Could you check a few things on this model? Use its own coordinates, in mm. Round coordinates to 2 decimals unless told otherwise and drop trailing zeros. Write each loop counter-clockwise with the first axis right and the second up, starting at its lowest first coordinate (ties: lowest second). Pieces come first, ordered by that corner, then holes. Notation, with made-up numbers: (26.5, 9.25) - (55.5, 9.25) arc R16 cw to (55.5, 17.25) - close; hole circle Ø5 at (2.5, 71). An arc over 180 degrees is marked (long way). Put each result on its own line as item: value.
from build123d import *

# Parameters (mm, degrees)
SKETCH1_R           = 3
SKETCH1_R_2         = 11.5
BOSS_EXTRUDE1_DEPTH = 4.7625


with BuildPart() as part:
    # Sketch1 → Boss-Extrude1 (new body)
    with BuildSketch(Plane.XY):
        Polygon((21.936631743, 65.154612456), (-64.58116939, 4.790688487), (-30.249253249, -44.416216862), (56.268547885, 15.947707107), align=None)
        with Locations(Location((-22.811758645, -2.646806117, 0), (0, 0, 180))):
            Circle(SKETCH1_R, mode=Mode.SUBTRACT)
        with Locations(Location((22.800025974, 29.176775421, 0), (0, 0, 180))):
            Circle(SKETCH1_R_2, mode=Mode.SUBTRACT)
    extrude(amount=BOSS_EXTRUDE1_DEPTH)


solid = part.part
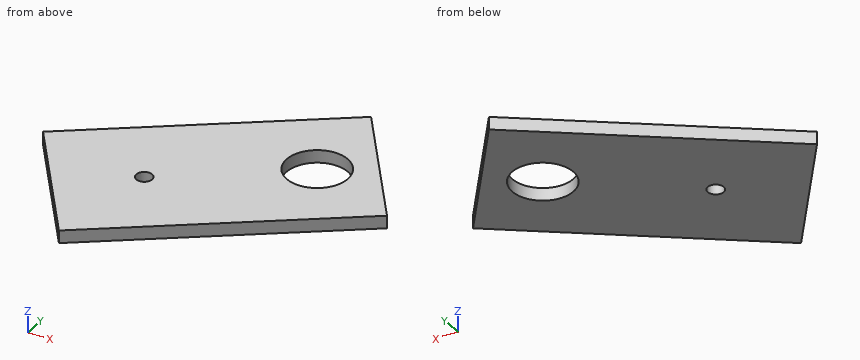
(1) Imagine slicing it at B-B, the plane x = 18. List the corners of the cut face in (y, z) for me, then the cut area to 3 significant figures.
Values found:
outline: (-10.75, 0) - (18.73, 0) - (18.73, 4.76) - (-10.75, 4.76) - close; (39.63, 0) - (62.41, 0) - (62.41, 4.76) - (39.63, 4.76) - close
area: 249 mm^2
(2) Imagine slicing it at D-D, the plane y = -18. List the corners of the cut face in (x, z) for me, then the cut area to 3 significant figures.
Values found:
outline: (-48.68, 0) - (7.61, 0) - (7.61, 4.76) - (-48.68, 4.76) - close
area: 268 mm^2
(3) I'm going to push flat-ended pins straight in: pin 1 (3.5 mm diameter, centred on x = -22.81, y = -2.65, fed in from +Z); pin 2 (2 mm diameter, centred on x = -45.5, z = 1, fed in from -Y); pin 3 (1.5 mm diameter, centred on y = 39.5, z = 4, fed in from -X); pin 4 (1 mm diameter, centred on y = 24, z = 4, fed in from -X). Where does each tip first touch, or does it pass through?
Values found:
pin 1: passes through
pin 2: stops at y = -23.99
pin 3: stops at x = -15.91
pin 4: stops at x = -37.77
(4) Imagine slicing it at A-A, the plane y = 38. List the corners of the cut face in (x, z) for me, then the cut area to 3 significant figures.
Values found:
outline: (-16.98, 0) - (15.42, 0) - (15.42, 4.76) - (-16.98, 4.76) - close; (30.18, 0) - (40.88, 0) - (40.88, 4.76) - (30.18, 4.76) - close
area: 205 mm^2
(5) Please list where these lines run through material, in increasing order: probe 1 along Y at (x, z) = (-22.5, 2.2); probe 2 along Y at (x, z) = (31.5, 1.5); probe 3 along X at (y, z) = (20, 3.65). Write a range as from..to.
Values found:
probe 1: y = -39.01..-5.63, 0.34..34.15
probe 2: y = -1.33..21.66, 36.7..51.45
probe 3: x = -42.78..15.87, 29.73..53.44
(6) Imagine slicing it at C-C, the plane z = 2.15. List the corners of the cut face in (x, y) for me.
Values found:
outline: (-64.58, 4.79) - (-30.25, -44.42) - (56.27, 15.95) - (21.94, 65.15) - close; hole circle Ø6 at (-22.81, -2.65); hole circle Ø23 at (22.8, 29.18)
